Design review of the part built by this model. Coordinates are the model's own, in mm. A direction names the side the tool comes from. Coordinates: 2 decimals unless noted, no trailing zeros. Write each loop counter-clockwise with the first axis right and the second up, starting at its lowest first coordinate (ties: lowest second). Pieces come first, ordered by that corner, then holes. Notation, with made-up numbers: M 66,77 L 112,77 A7 cw 112,82 Z; hole C 21.25,-31 d9. An arc over 180 degrees is marked long. One line per question, with ' | ' between items.
from build123d import *

# Parameters (mm, degrees)
SKETCH_1_W          = 65
SKETCH_1_H          = 40
EXTRUDE_1_DEPTH     = 2
SKETCH_2_R          = 2
CUT_EXTRUDE_1_DEPTH = 77.347887987
SKETCH_3_W          = 47
SKETCH_3_H          = 43
EXTRUDE_2_DEPTH     = 2
RIB_1_REACH         = 84.225
SKETCH_5_WALL_W     = 223.835267426
SKETCH_5_WALL_H     = 2
RIB_START           = -2
RIB_2_DEPTH         = 2
SKETCH_7_R          = 11.5
SKETCH_7_R_2        = 1.6
CUT_EXTRUDE_2_DEPTH = 88.715449038
FILLET_1_R          = 3


# Read off the part's stored shape, not the designer's step: the rib step
with BuildPart() as part:
    # Sketch 1 → Extrude 1 (new body)
    with BuildSketch(Plane(origin=(0, 0, 0), x_dir=(1, 0, 0), z_dir=(0, 1, 0))):
        with Locations((32.5, 20)):
            Rectangle(SKETCH_1_W, SKETCH_1_H)
    extrude(amount=EXTRUDE_1_DEPTH)

    # Sketch 2 → Cut-Extrude 1 (cut, through all)
    with BuildSketch(Plane(origin=(0, 2, 0), x_dir=(1, 0, 0), z_dir=(0, 1, 0))):
        with Locations(Location((5.7, 5, 0), (0, 0, 270))):
            Circle(SKETCH_2_R)
        with Locations(Location((5.7, 20, 0), (0, 0, 270))):
            Circle(SKETCH_2_R)
        with Locations(Location((5.7, 35, 0), (0, 0, 270))):
            Circle(SKETCH_2_R)
        with Locations(Location((59.3, 5, 0), (0, 0, 90))):
            Circle(SKETCH_2_R)
        with Locations(Location((59.3, 20, 0), (0, 0, 90))):
            Circle(SKETCH_2_R)
        with Locations(Location((59.3, 35, 0), (0, 0, 90))):
            Circle(SKETCH_2_R)
    extrude(amount=-CUT_EXTRUDE_1_DEPTH, mode=Mode.SUBTRACT)

    # Sketch 3 → Extrude 2 (add)
    with BuildSketch(Plane.XY):
        with Locations((32.5, 23.5)):
            Rectangle(SKETCH_3_W, SKETCH_3_H)
    extrude(amount=-EXTRUDE_2_DEPTH)

    # Sketch 5 wall → Rib 1 (add, up to next)
    with BuildSketch(Plane(origin=(9, 23.5, -21), x_dir=(0, 0.749329085481, 0.662197796472), z_dir=(0, 0.662197796472, -0.749329085481)), mode=Mode.PRIVATE) as rib_1_sk1:
        with Locations((0, 1)):
            Rectangle(SKETCH_5_WALL_W, SKETCH_5_WALL_H)
    rib_1_tool1 = extrude(rib_1_sk1.sketch, amount=-RIB_1_REACH, mode=Mode.PRIVATE) - part.part
    add(rib_1_tool1.solids().sort_by_distance((9, 23.5, -21))[0])

    # Rib 2 outline → Rib 2 (add)
    with BuildSketch(Plane(origin=(56, 0, 0), x_dir=(0, 0, -1), z_dir=(1, 0, 0)).offset(RIB_START)):
        Polygon((40, 2), (2, 45), (2, 2), align=None)
    extrude(amount=RIB_2_DEPTH)

    # Sketch 7 → Cut-Extrude 2 (cut, through all)
    with BuildSketch(Plane(origin=(0, 0, -2), x_dir=(-1, 0, 0), z_dir=(0, 0, -1))):
        with Locations((-32.5, 23.5)):
            Circle(SKETCH_7_R)
        with Locations((-48.15, 7.85)):
            Circle(SKETCH_7_R_2)
        with Locations((-16.85, 7.85)):
            Circle(SKETCH_7_R_2)
        with Locations((-16.85, 39.15)):
            Circle(SKETCH_7_R_2)
        with Locations((-48.15, 39.15)):
            Circle(SKETCH_7_R_2)
    extrude(amount=-CUT_EXTRUDE_2_DEPTH, mode=Mode.SUBTRACT)

    # Fillet 1
    fillet_1_edges = [part.edges().sort_by_distance(p)[0] for p in [
        (0, 1, -40),
        (65, 1, -40),
        (65, 1, 0),
        (0, 1, 0),
    ]]
    fillet(fillet_1_edges, radius=FILLET_1_R)


solid = part.part
1. Take a section at B-B (y = 23.5). Write out the cut boundary in (x, z), then the cut area to 3 significant figures.
Answer sheet:
outline: M 9,-21 L 11,-21 L 11,-2 L 21,-2 L 21,0 L 9,0 Z; M 44,-2 L 54,-2 L 54,-21 L 56,-21 L 56,0 L 44,0 Z | area: 124 mm^2
2. Tool access review of faces 4 (the face through (54, 14, -12)), 5 (the face through (9, 16, -12)), 6 (the face through (56, 19, -15)), 7 (the face through (6.301, 1.014, -33.092)): name each direction out of +Z, -Z, +X, -X, +Y, -Y from which nothing blocks a thin tool from reaching the whole face with its end or side.
Answer sheet:
face 4: -Z, +Y | face 5: +Z, -Z, -X, +Y | face 6: +Z, -Z, +X, +Y | face 7: +Y, -Y
3. Draft analysis for pull direction Z (two halves, no side actions). For faces 1 (the face through (60.5, 1, -3.4)), 2 (the face through (10.014, 23.199, -21.266)), 3 (the face through (32, 0, -20)), state which applies: pulls with the +Z half, pulls with the -Z half, needs draft (parallel to the pull), parting line crosses it, or undercut.
Answer sheet:
face 1: undercut | face 2: pulls with the -Z half | face 3: needs draft
4. To check wall thickness, follow line 1 along X through (y, z) = (1.05, -35); line 2 along X through (y, z) = (15, -18.5); line 3 along Y through (x, z) = (48, -1). State the ranges of each line that lie inside material, in increasing order. Write a range as [from, to].
Answer sheet:
line 1: [0, 3.7], [7.7, 57.3], [61.3, 65] | line 2: [9, 11], [54, 56] | line 3: [0, 6.26], [9.44, 37.56], [40.74, 45]
5. Take a section at D-D (y = 7). Write out the cut boundary in (x, z), then the cut area to 3 significant figures.
Answer sheet:
outline: M 9,-35.58 L 11,-35.58 L 11,-2 L 15.49,-2 L 15.49,0 L 9,0 Z; M 18.21,-2 L 46.79,-2 L 46.79,0 L 18.21,0 Z; M 49.51,-2 L 54,-2 L 54,-35.58 L 56,-35.58 L 56,0 L 49.51,0 Z | area: 217 mm^2
6. Take a section at C-C (x = 16.85). Write out the cut boundary in (y, z), then the cut area to 3 significant figures.
Answer sheet:
outline: M 0,-40 L 2,-40 L 2,-2 L 6.25,-2 L 6.25,0 L 0,0 Z; M 9.45,-2 L 37.55,-2 L 37.55,0 L 9.45,0 Z; M 40.75,-2 L 45,-2 L 45,0 L 40.75,0 Z | area: 153 mm^2
7. Insertion check: pin 1 Ø1.5 at (x, z) = (43.5, -24) entering from +Y; pin 2 Ø2.5 at (x, y) = (16.85, 7.85) entering from -Z; pin 3 Ø1.5 at (y, z) = (30, -4) entering from -X. Each pin has a flat end and moves straight along its axis. Give the tip position at first contact, or say it passes through.
Answer sheet:
pin 1: y = 2 | pin 2: through | pin 3: x = 9
8. Take a section at A-A (x = 32.5). Write out the cut boundary in (y, z).
Answer sheet:
outline: M 0,-40 L 2,-40 L 2,-2 L 12,-2 L 12,0 L 0,0 Z; M 35,-2 L 45,-2 L 45,0 L 35,0 Z
